Verification items for the finished model (mm, model axes). Face numbers are marked on the shaded views. A direction names the side the tool comes from. Give positions to 0.01 mm unless a question says otherwise; leave off trailing zeros. Write each loop counter-clockwise with the first axis right and the second up, starting at its lowest first coordinate (ties: lowest second). Pieces come first, ordered by that corner, then holes. Notation, with made-up numbers: (22.5, -20.75) - (68.5, -20.75) arc R33 cw to (68.5, 18.25) - close; hole circle Ø9 at (57.5, 5.25). An arc over 180 degrees is marked (long way). Put each result on its own line as item: value.
from build123d import *

# Parameters (mm, degrees)
SUPERFICIE_EXTRUIR1_1_DEPTH = 40
DAR_ESPESOR1_T1             = 3
CROQUIS2_R                  = 5
EXTRUIR1_DEPTH              = 23
CROQUIS3_R                  = 5
EXTRUIR2_DEPTH              = 20


with BuildPart() as body_1:
    # Superficie-Extruir1: a surface, the sketch's curves swept straight by 40 mm
    with BuildLine(Plane.XY, mode=Mode.PRIVATE) as superficie_extruir1_1_path:
        Line((0, -70), (0, 0))
        Line((0, 0), (-50, 0))
    superficie_extruir1_1 = Shell.extrude(superficie_extruir1_1_path.wire(), (0 * SUPERFICIE_EXTRUIR1_1_DEPTH, 0 * SUPERFICIE_EXTRUIR1_1_DEPTH, 1 * SUPERFICIE_EXTRUIR1_1_DEPTH))
    add(Solid.thicken(superficie_extruir1_1, DAR_ESPESOR1_T1))

    # Croquis2 → Extruir1 (add)
    with BuildSketch(Plane(origin=(0, 0, 0), x_dir=(1, 0, 0), z_dir=(0, 1, 0))):
        with Locations(Location((-35, -20, 0), (0, 0, 180))):
            Circle(CROQUIS2_R)
    extrude(amount=-EXTRUIR1_DEPTH)

    # Croquis3 → Extruir2 (cut)
    with BuildSketch(Plane.ZY.offset(3)):
        with Locations(Location((20, -56.5, 0), (0, 0, 270))):
            Circle(CROQUIS3_R)
        with Locations(Location((20, -16.5, 0), (0, 0, 90))):
            Circle(CROQUIS3_R)
    extrude(amount=-EXTRUIR2_DEPTH, mode=Mode.SUBTRACT)


solid = body_1.part
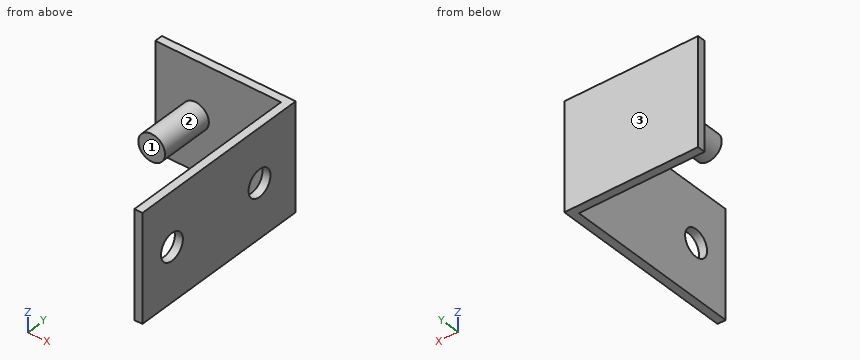
Q1. Section check D-D, the plane x = -35. Record the cut outline in (y, z), plus the area to 3 significant figures.
Answers follow:
outline: (-23, 15) - (-3, 15) - (-3, 0) - (0, 0) - (0, 40) - (-3, 40) - (-3, 25) - (-23, 25) - close
area: 320 mm2
Q2. Scan lines: line 1 along Z through (x, y) = (-1.05, -16.5); line 2 along Y through (x, z) = (-8, 22). Record each from-to range of solid material in increasing order.
Answers follow:
line 1: z = 0 to 15, 25 to 40
line 2: y = -3 to 0
Q3. Section check C-C, the plane y = -16.5. Record the cut outline in (x, z).
Answers follow:
outline: circle Ø10 at (-35, 20); (-3, 0) - (0, 0) - (0, 15) - (-3, 15) - close; (-3, 25) - (0, 25) - (0, 40) - (-3, 40) - close
Q4. Section check B-B, the plane y = -56.5. Record the cut outline in (x, z).
Answers follow:
outline: (-3, 0) - (0, 0) - (0, 15) - (-3, 15) - close; (-3, 25) - (0, 25) - (0, 40) - (-3, 40) - close
Q5. Go/stop test with flat-tipped pins: pin 1 Ø11.5 at (y, z) = (-16.5, 20) entering from -X; pin 2 Ø20 at (x, z) = (-16, 13) entering from -Y; pin 3 Ø10 at (x, z) = (-32, 20.5) entering from -Y. Record where each tip stops, or that it passes through.
Answers follow:
pin 1: stops at x = -40
pin 2: stops at y = -3
pin 3: stops at y = -23
Q6. Section check A-A, the plane z = 20. Record the cut outline in (x, y).
Answers follow:
outline: (-50, -3) - (-40, -3) - (-40, -23) - (-30, -23) - (-30, -3) - (-3, -3) - (-3, -11.5) - (0, -11.5) - (0, 0) - (-50, 0) - close; (-3, -70) - (0, -70) - (0, -61.5) - (-3, -61.5) - close; (-3, -51.5) - (0, -51.5) - (0, -21.5) - (-3, -21.5) - close
Q7. Set-up check for the marked faces 1, 2 and 3: record each of +Z, -Z, +X, -X, +Y, -Y from which the full face is reachable in a straight line by a thin tool's end or side.
Answers follow:
face 1: +Z, -Z, -X, -Y
face 2: -Y
face 3: +Z, -Z, +X, -X, +Y
